Source: CAD feature listing. Evaluate the final solid. Frame: model axes, mm. A direction names the side the tool comes from. Round coordinates to 2 decimals unless told otherwise and drop trailing zeros. Loops run counter-clockwise (first coordinate to the right, second up) from the corner with the lowest first, then second, coordinate; pieces in that order, holes last.
(1) Section A-A, the plane z = 19. Return the cut outline in (x, y).
(2) Material intervals for probe 1 along Y at (x, z) = (-8, 13.5); probe 2 along Z at (x, y) = (1, -30.5); probe 3 along Y at (x, z) = (6.5, 9), sorted ascending.
(3) First-contact query: pin 1 Ø4.5 at (y, z) = (0, 9.5) entering from +X; pin 2 Ø5 at (x, y) = (4.5, 6.5) entering from +Z; pin 3 Ø2 at (x, y) = (-0.5, 0.5) entering from +Z; pin 4 Ø10 at (y, z) = (-27.5, 9) entering from +X. Flat tips, straight axial feed; report the tip coordinate or a pass-through.
(4) Set-up query: faces 4 (the flat face through (-8, 16.881, 16)), 5 (the flat face through (-12.975, 0, 9)), 6 (the flat face through (-1, 0, 10.9)), 7 (the flat face through (11.928, 0, 9)). Return all of +Z, -Z, +X, -X, +Y, -Y with unobstructed straight access to the full face (end or side cutting, diameter ignored); none if empty.
(5) Mould query, pull axis X, two halves, no side actions, for faces 1 (the flat face through (2, -17.019, 13)), 2 (the cylindrical face through (9.62, -0.31, 18.54)), 3 (the flat face through (-2.793, -0.306, 17.242)). Classes: pulls with the +X half, pulls with the -X half, needs draft (parallel to the pull), parting line crosses it, or undercut.
(6) Section D-D, the plane y = -21. Return the cut outline in (x, z), plus the area to 3 significant figures.
(7) Section B-B, the plane y = 0.5. Return the cut outline in (x, z).
(8) Section C-C, the plane x = 6. Return the cut outline in (y, z).
```python
from build123d import *

# Parameters (mm, degrees)
F0_W     = 37.984425202
F0_H     = 123.9991616458
F0_W_2   = 24.9025691301
F0_H_2   = 33.8271874934
F1_DEPTH = 6.6
F2_DEPTH = 10.9
F4_DEPTH = 33.9


with BuildPart() as f1:
    # F0 (on Top) → F1 (new body)
    with BuildSketch(Plane.XY):
        with Locations((-0.5247322842, 0.4318514839)):
            Rectangle(F0_W, F0_H)
        with Locations((-0.5233194679, -0.1052441075)):
            Rectangle(F0_W_2, F0_H_2, mode=Mode.SUBTRACT)
    extrude(amount=F1_DEPTH)

    # F0 (on Top) → F2 (join)
    with BuildSketch(Plane.XY):
        with Locations((-0.5233194679, -0.1052441075)):
            Rectangle(F0_W_2, F0_H_2)
    extrude(amount=F2_DEPTH)

    # F3 (on face) → F4 (join)
    with BuildSketch(Plane.XZ.offset(17.0188378543)):
        with BuildLine():
            Line((3.2664190512, 23.7103309482), (0.6797150322, 10.9))
            Line((0.6797150322, 10.9), (11.9279650971, 10.9))
            ThreePointArc((11.9279650971, 10.9), (9.5593663419, 18.6318652166), (3.2664190512, 23.7103309482))
        make_face()
        with BuildLine():
            Line((-1.8759769267, 10.9), (-3.7359872367, 23.7637832761))
            ThreePointArc((-3.7359872367, 23.7637832761), (-10.4256426154, 18.8187903193), (-12.9746040329, 10.9))
            Line((-12.9746040329, 10.9), (-1.8759769267, 10.9))
        make_face()
    extrude(amount=-F4_DEPTH)


solid = f1.part
```
Output values:
1. outline: (-10.29, -17.02) - (-3.05, -17.02) - (-3.05, 16.88) - (-10.29, 16.88) - close; (2.32, -17.02) - (9.3, -17.02) - (9.3, 16.88) - (2.32, 16.88) - close
2. probe 1: y = -17.02 to 16.88
2. probe 2: z = 0 to 6.6
2. probe 3: y = -17.02 to 16.81
3. pin 1: stops at x = 11.93
3. pin 2: stops at z = 23.71
3. pin 3: stops at z = 10.9
3. pin 4: stops at x = 18.47
4. face 4: +Z, +X, -X, +Y
4. face 5: +Z, -X, +Y, -Y
4. face 6: +Z, +Y, -Y
4. face 7: +Z, +X, +Y, -Y
5. face 1: needs draft
5. face 2: pulls with the +X half
5. face 3: undercut
6. outline: (-19.52, 0) - (18.47, 0) - (18.47, 6.6) - (-19.52, 6.6) - close
6. area: 251 mm2
7. outline: (-19.52, 0) - (18.47, 0) - (18.47, 6.6) - (11.93, 6.6) - (11.93, 10.9) arc R13.8 ccw to (3.27, 23.71) - (0.68, 10.9) - (-1.88, 10.9) - (-3.74, 23.76) arc R13.58 ccw to (-12.97, 10.9) - (-12.97, 6.6) - (-19.52, 6.6) - close
8. outline: (-61.57, 0) - (62.43, 0) - (62.43, 6.6) - (16.81, 6.6) - (16.81, 10.9) - (16.88, 10.9) - (16.88, 22.24) - (-17.02, 22.24) - (-17.02, 6.6) - (-61.57, 6.6) - close
